Work out the finished part from the listing and answer in its coordinate system (mm). A direction names the side the tool comes from. Coordinates: 2 decimals unless noted, no trailing zeros. Loops run counter-clockwise (first coordinate to the right, second up) from the corner with the lowest first, then second, coordinate; pieces in that order, holes last.
```python
from build123d import *

# Parameters (mm, degrees)
F1_DEPTH = 7.62
F2_SIZE  = 5.08
F3_W     = 39.5873952657
F3_H     = 5.6298854761
F4_DEPTH = 31.242
F6_DEPTH = 34.798


with BuildPart() as f1:
    # F0 (on Top) → F1 (new body)
    with BuildSketch(Plane.XY):
        Polygon((-76.5226408839, 20.2266871929), (-76.5226408839, 0), (59.1854825616, 0), (59.1854825616, 18.4331871569), (18.3335505426, 18.4331871569), (15.344383195, 24.4115199894), (4.1848318651, 27.7992393821), (4.1848318651, 60.2815076709), (-21.5219929814, 60.2815076709), (-21.5219929814, 27.7992393821), (-31.2866009772, 25.4079084843), (-33.8772125542, 20.2266871929), align=None)
    extrude(amount=F1_DEPTH)

    # F2
    f2_edges = [f1.edges().sort_by_distance(p)[0] for p in [
        (-26.404297, 26.603574, 7.62),
        (-32.581907, 22.817298, 7.62),
        (9.764608, 26.10538, 7.62),
        (16.838967, 21.422354, 7.62),
        (59.185483, 9.216594, 0),
        (-76.522641, 10.113344, 0),
        (-8.668581, 60.281508, 0),
    ]]
    chamfer(f2_edges, length=F2_SIZE)

    # F3 (on face) → F4 (join)
    with BuildSketch(Plane.XY.offset(7.62)):
        with Locations((-10.2241346613, 2.814942738)):
            Rectangle(F3_W, F3_H)
    extrude(amount=F4_DEPTH)

    # F5 (on face) → F6 (join)
    with BuildSketch(Plane(origin=(0, 5.6298854761, 0), x_dir=(-1, 0, 0), z_dir=(0, 1, 0))):
        Polygon((-4.6187778935, 25.9514674544), (-4.6187778935, 7.62), (0, 7.62), (0, 23.0201836675), (4.759604577, 29.3508209288), (15.9931536764, 29.3508209288), (19.8779646307, 25.9514674544), (19.8779646307, 7.62), (23.7236581743, 7.62), (23.7236581743, 33.3591811359), (15.9931536764, 38.862), (4.759604577, 38.862), align=None)
        Polygon((0, 23.0201836675), (0, 7.62), (19.8779646307, 7.62), (19.8779646307, 25.9514674544), (15.9931536764, 29.3508209288), (4.759604577, 29.3508209288), align=None)
    extrude(amount=F6_DEPTH)


solid = f1.part
```
1. A cutting plane is placed at D-D, the plane y = 36. Give the vertices of the cut face in (x, z).
2. A cutting plane is placed at B-B, the plane z = 11. Give the vertices of the cut face in (x, y).
3. A cutting plane is placed at C-C, the plane x = -37. Give the vertices of the cut face in (y, z).
4. Determine the mould class of faces 4 (the flat face through (15.06, 20.48, 4.55)), 5 (the flat face through (-25.723, 24.119, 5.116)), 6 (the flat face through (4.619, 23, 17)) for opening direction Z: released by +Z, released by -Z, zero draft, split by the parting line, or undercut.
5. Each of these flat-tipped pins is pushed along its axis until it touches: P1, Ø10, axis at x = -15, y = 54, coming from the +Z side; P2, Ø15.5, axis at x = -25, z = 17, coming from the +Y side; P3, Ø8.5, axis at y = 45, z = 5.5, coming from the +X side. Where does it stop, or does it pass through?
6. A cutting plane is placed at A-A, the plane y = 9. Give the vertices of the cut face in (x, z), then the cut area to 3 significant figures.
7. For faces 1 (the flat face through (9.57, 3, 23)), 2 (the flat face through (-23.724, 23, 20)), 3 (the flat face through (-9, 50, 7.62)), determine the directions among +Z, -Z, +X, -X, +Y, -Y from which every point of the face is accessible in a straight line to the end or side of a thin tool.
8. Straight lines are drawn through the part: probe 1 along Y at (x, z) = (-17, 14); probe 2 along X at (y, z) = (5, 10.5); probe 3 along X at (y, z) = (10, 17.5). For each, find the intervals that lie inside material, in ascending order.
Answers below:
1. outline: (-23.72, 7.62) - (-21.52, 7.62) - (-21.52, 0) - (4.18, 0) - (4.18, 7.62) - (4.62, 7.62) - (4.62, 25.95) - (-4.76, 38.86) - (-15.99, 38.86) - (-23.72, 33.36) - close
2. outline: (-30.02, 0) - (9.57, 0) - (9.57, 5.63) - (4.62, 5.63) - (4.62, 40.43) - (-23.72, 40.43) - (-23.72, 5.63) - (-30.02, 5.63) - close
3. outline: (0, 0) - (20.23, 0) - (20.23, 7.62) - (0, 7.62) - close
4. face 4: released by +Z
4. face 5: undercut
4. face 6: zero draft
5. P1: stops at z = 7.62
5. P2: stops at y = 40.43
5. P3: stops at x = 4.18
6. outline: (-76.52, 5.08) - (-71.44, 0) - (54.11, 0) - (59.19, 5.08) - (59.19, 7.62) - (4.62, 7.62) - (4.62, 25.95) - (-4.76, 38.86) - (-15.99, 38.86) - (-23.72, 33.36) - (-23.72, 7.62) - (-76.52, 7.62) - close
6. area: 1,810 mm2
7. face 1: +Z, +X, +Y, -Y
7. face 2: +Z, -X, +Y
7. face 3: +Z, +X, -X, +Y
8. probe 1: y = 0 to 40.43
8. probe 2: x = -30.02 to 9.57
8. probe 3: x = -23.72 to 4.62
